Verification items for this drawing (mm, ordinates from the low corner). A direction names the side the tool comes from. Coordinates: 2 decimals unless noted, no trailing zeros. Order: outer loops, then holes, each group sorted by start corner. A loop starts at its lowest first (then second) coordinate and runs counter-clockwise, first axis right, second up. Notation, with made-up numbers: M 83.25,-35.5 L 97.25,-35.5 A6 ccw 97.25,-27.5 Z; hole C -1,54.5 d9. An arc over 180 degrees is marked long. Use CSV: the item, a comma, the result in double quotes. Start each with the question number.
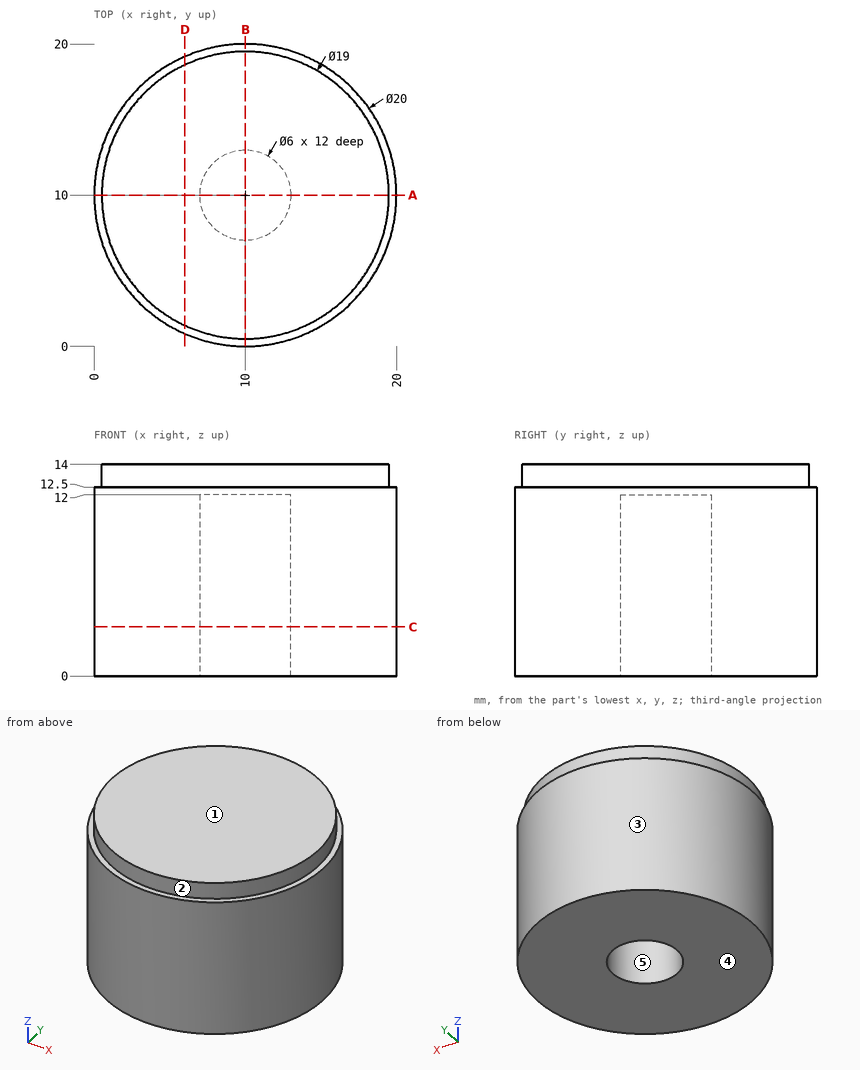
1) Material ranges on line 1 along Y through (x, z) = (10, 6.25); line 2 along X through (y, z) = (9.75, 10.75); line 3 along Y through (x, z) = (4.25, 10), recorded low to high.
2) Draft check along Y on the marked faces 3, 4 and 5. Enter one of: +Y half, -Y half, draft (parallel to the pull), parting line (faces both ways), or undercut.
3) Gauge pin test, flat ends, axial feed: P1, Ø10, axis at x = 12, y = 2.5, coming from the -Z side; P2, Ø3, axis at y = 7.5, z = 5, coming from the +X side; P3, Ø4, axis at x = 6, z = 3.5, coming from the -Y side. Record the tip position at first contact, or that the pin passes through.
4) Section check C-C on z = 3.25. Record the boundary of the cut face in (x, y).
5) Section check D-D on x = 6. Record the boundary of the cut face in (y, z), then the cut area to 3 significant figures.
6) Set-up check for the marked faces 1 and 2: record each of +Z, -Z, +X, -X, +Y, -Y from which the full face is reachable in a straight line by a thin tool's end or side.
7) Section check A-A on y = 10. Record the boundary of the cut face in (x, z).
Results are:
1,line 1,"y = 0 to 7, 13 to 20"
1,line 2,"x = 0 to 7.01, 12.99 to 20"
1,line 3,"y = 1.82 to 18.18"
2,face 3,"parting line"
2,face 4,"draft"
2,face 5,"undercut"
3,P1,"stops at z = 0"
3,P2,"stops at x = 19.95"
3,P3,"stops at y = 0.2"
4,outline,"C 10,10 d20; hole C 10,10 d6"
5,outline,"M 0.83,0 L 19.17,0 L 19.17,12.5 L 18.62,12.5 L 18.62,14 L 1.38,14 L 1.38,12.5 L 0.83,12.5 Z"
5,area,"255 mm²"
6,face 1,"+Z, +X, -X, +Y, -Y"
6,face 2,"+Z"
7,outline,"M 0,0 L 7,0 L 7,12 L 13,12 L 13,0 L 20,0 L 20,12.5 L 19.5,12.5 L 19.5,14 L 0.5,14 L 0.5,12.5 L 0,12.5 Z"
